```python
from build123d import *

# Parameters (mm, degrees)
SM_BASE_FLANGE_1_DEPTH = 1


# Sheet-metal steps are written as plain solids
with BuildPart() as part:
    # Sketch 1 → Базовая кромка1 (new body)
    with BuildSketch(Plane.XY):
        with BuildLine():
            Line((89.221000297, -66.773952096), (89.221000297, -28.520742394))
            ThreePointArc((89.221000297, -28.520742394), (90.685466391, -24.985208488), (94.221000297, -23.520742394))
            Line((94.221000297, -23.520742394), (128.329321471, -23.520742394))
            ThreePointArc((128.329321471, -23.520742394), (131.864855377, -24.985208488), (133.329321471, -28.520742394))
            Line((133.329321471, -28.520742394), (133.329321471, -66.773952096))
            Line((133.329321471, -66.773952096), (204.25, -66.773952096))
            ThreePointArc((204.25, -66.773952096), (205.664213562, -66.188165658), (206.25, -64.773952096))
            Line((206.25, -64.773952096), (206.25, 41.226047904))
            ThreePointArc((206.25, 41.226047904), (205.664213562, 42.640261467), (204.25, 43.226047904))
            Line((204.25, 43.226047904), (-66.75, 43.226047904))
            ThreePointArc((-66.75, 43.226047904), (-68.164213562, 42.640261467), (-68.75, 41.226047904))
            Line((-68.75, 41.226047904), (-68.75, -64.773952096))
            ThreePointArc((-68.75, -64.773952096), (-68.164213562, -66.188165658), (-66.75, -66.773952096))
            Line((-66.75, -66.773952096), (89.221000297, -66.773952096))
        make_face()
    extrude(amount=-SM_BASE_FLANGE_1_DEPTH)


solid = part.part
```
Model file for the job. Use its own axes, mm. A direction names the side the tool comes from. Coordinates: 2 decimals unless noted, no trailing zeros. Loops run counter-clockwise (first coordinate to the right, second up) from the corner with the lowest first, then second, coordinate; pieces in that order, holes last. Notation, with made-up numbers: (-35, 63.25) - (-31, 63.25) arc R24 ccw to (-31, 83.25) - close; hole circle Ø3 at (-6.5, 13). An arc over 180 degrees is marked (long way). Write item = value, one per line. Start each with the question number.
Item 1: 3-axis set-ups, long thin cutter, end or side, ignore diameter. For faces 1 (the face through (131.83, -24.95, -0.49)), 2 (the face through (67, -11, -1)): which of +Z, -Z, +X, -X, +Y, -Y reach the whole face in a straight line?
Item 2: Saw through at C-C, the plane x = 107. List the corners of the cut face in (y, z), then the cut area to 3 significant figures.
Item 3: Wall check: probe 1 along X at (y, z) = (-58, -0.5); probe 2 along Y at (x, z) = (109, -0.7); probe 3 along X at (y, z) = (-24.5, -0.7). Give the ranges that are in metal, low to high. Write a range as [from, to].
Item 4: Saw through at A-A, the plane y = -54. List the corners of the cut face in (x, z).
Item 5: Drop a flat-ended pin along its axis: pin 1 Ø0.5 at (x, z) = (111, -0.5) entering from -Y. Give the stop position or say it passes through.
Item 6: Saw through at B-B, the plane z = -0.45. List the corners of the cut face in (x, y).
Item 7: Pull direction X, two halves, no side cores. Call faces 3 (the face through (90.65, -25.02, -0.49)), 4 (the face through (67, -11, 0)): +X half, -X half, draft (parallel to the pull), parting line (faces both ways), or undercut.
Answers:
q1.face_1 = +Z, -Z, -Y
q1.face_2 = -Z, +X, -X, +Y, -Y
q2.outline = (-23.52, -1) - (43.23, -1) - (43.23, 0) - (-23.52, 0) - close
q2.area = 66.7 mm2
q3.probe_1 = [-68.75, 89.22], [133.33, 206.25]
q3.probe_2 = [-23.52, 43.23]
q3.probe_3 = [-68.75, 91.25], [131.3, 206.25]
q4.outline = (-68.75, -1) - (89.22, -1) - (89.22, 0) - (-68.75, 0) - close; (133.33, -1) - (206.25, -1) - (206.25, 0) - (133.33, 0) - close
q5.pin_1 = -23.52
q6.outline = (-68.75, -64.77) arc R2 ccw to (-66.75, -66.77) - (89.22, -66.77) - (89.22, -28.52) arc R5 cw to (94.22, -23.52) - (128.33, -23.52) arc R5 cw to (133.33, -28.52) - (133.33, -66.77) - (204.25, -66.77) arc R2 ccw to (206.25, -64.77) - (206.25, 41.23) arc R2 ccw to (204.25, 43.23) - (-66.75, 43.23) arc R2 ccw to (-68.75, 41.23) - close
q7.face_3 = undercut
q7.face_4 = draft
